The listing builds one solid part. Answer for the finished solid, in the listing's coordinates (mm). Coordinates: 2 decimals unless noted, no trailing zeros. Order: outer loops, then holes, each group sorted by start corner. A loop starts at its lowest first (then second) coordinate and runs counter-clockwise, first axis right, second up.
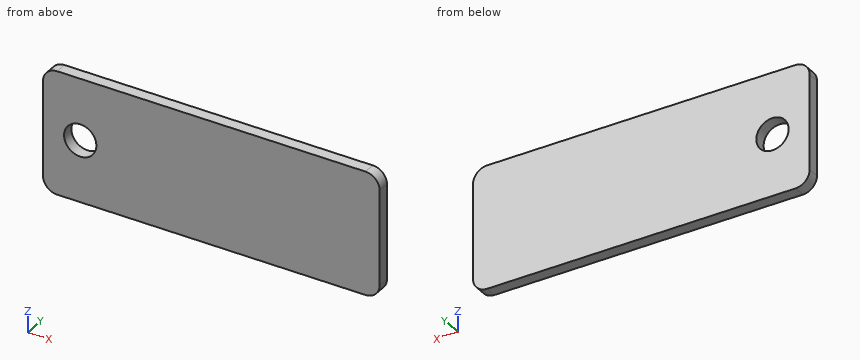
```python
from build123d import *

# Parameters (mm, degrees)
F0_R     = 3.40703
F1_DEPTH = 2.5


with BuildPart() as f1:
    # F0 (on Front) → F1 (new body)
    with BuildSketch(Plane.XZ):
        with BuildLine():
            Line((60.151453, 13), (-4.848547, 13))
            ThreePointArc((-4.848547, 13), (-6.969868, 12.12132), (-7.848547, 10))
            Line((-7.848547, 10), (-7.848547, -10))
            ThreePointArc((-7.848547, -10), (-6.969868, -12.12132), (-4.848547, -13))
            Line((-4.848547, -13), (60.151453, -13))
            ThreePointArc((60.151453, -13), (62.272773, -12.12132), (63.151453, -10))
            Line((63.151453, -10), (63.151453, 10))
            ThreePointArc((63.151453, 10), (62.272773, 12.12132), (60.151453, 13))
        make_face()
        Circle(F0_R, mode=Mode.SUBTRACT)
    extrude(amount=F1_DEPTH)


solid = f1.part
```
(1) This flat-tipped pin is pushed along its axis until it touches: pin 1 Ø4 at (x, z) = (0, 0) entering from -Y. Where does it stop, or does it pass through?
(2) Find section A-A (x = 0). Write down the section's boundary in (y, z).
(3) Consider line 1 (Z direction, x = 0, y = -1.9); line 2 (X direction, y = -2.1, z = -0.25); line 3 (X direction, y = -0.85, z = 10.25). Determine where each line is inside the solid, lowest interval first.
(4) Find section B-B (z = -2). Write down the section's boundary in (x, y), and give its area (3 significant figures).
Findings below:
1. pin 1: passes through
2. outline: (-2.5, -13) - (0, -13) - (0, -3.41) - (-2.5, -3.41) - close; (-2.5, 3.41) - (0, 3.41) - (0, 13) - (-2.5, 13) - close
3. line 1: z = -13 to -3.41, 3.41 to 13
3. line 2: x = -7.85 to -3.4, 3.4 to 63.15
3. line 3: x = -7.84 to 63.14
4. outline: (-7.85, -2.5) - (-2.76, -2.5) - (-2.76, 0) - (-7.85, 0) - close; (2.76, -2.5) - (63.15, -2.5) - (63.15, 0) - (2.76, 0) - close
4. area: 164 mm2
